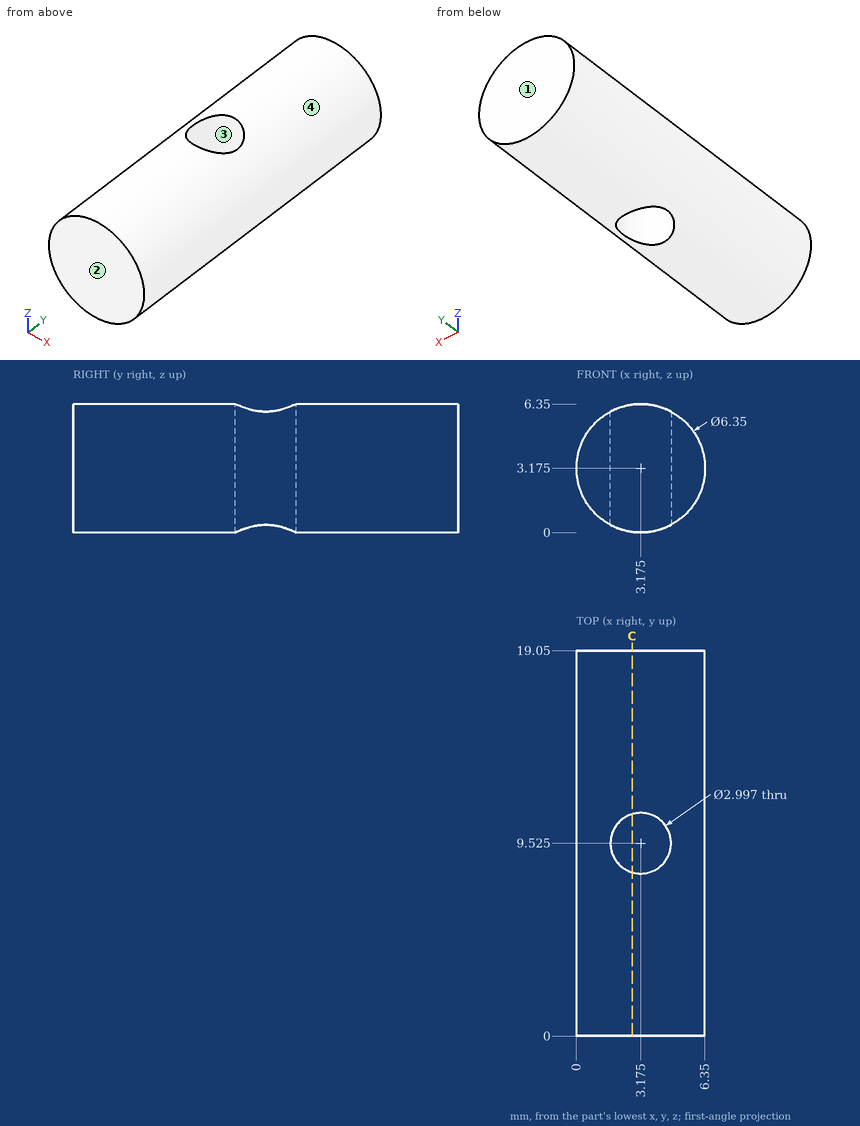
The figure shows three views and two pictorial views of one solid part (mm, origin at its lowest corner). Answer the questions. Coordinates: 2 decimals unless noted, no trailing zeros. Order: outer loops, then holes, each group sorted by start corner. A loop starts at its lowest first (then second) coordinate and runs counter-clockwise, first axis right, second up. Notation, with made-up numbers: M 1.5,55.25 L 28.5,55.25 A13 ccw 28.5,71.25 Z; hole C 80,-25 d1. An arc over 180 degrees is marked long. Use CSV: the item, a comma, the result in double quotes.
1) Determine the mould class of the marked faces 1, 2, 3 and 4 for opening direction Y: released by +Y, released by -Y, zero draft, split by the parting line, or undercut.
Worked out:
face 1,"released by +Y"
face 2,"released by -Y"
face 3,"undercut"
face 4,"zero draft"
2) Consider line 1 (Y direction, x = 3.75, z = 2.25); line 2 (X direction, y = 10.5, z = 2) (1 decimal); line 3 (Y direction, x = 4.25, z = 3.5). Determine where each line is inside the solid, lowest interval first. Write a range as [from, to].
Worked out:
line 1,"y = [0, 8.14], [10.91, 19.05]"
line 2,"x = [0.2, 2], [4.3, 6.1]"
line 3,"y = [0, 8.48], [10.57, 19.05]"
3) Section C-C on x = 2.75 is taken. Write down the section's boundary in (y, z), plus the area to 3 significant figures.
Worked out:
outline,"M 0,0.03 L 8.09,0.03 L 8.09,6.32 L 0,6.32 Z; M 10.96,0.03 L 19.05,0.03 L 19.05,6.32 L 10.96,6.32 Z"
area,"102 mm^2"
4) A flat-ended cylindrical pin translates along its axis: pin 1 Ø2 at (y, z) = (16, 0.5) entering from -X. Find the tip coordinate at first contact, or state that the pin passes through.
Worked out:
pin 1,"stops at x = 0.48"
